Could you check a few things on this model? Use its own coordinates, in mm. A direction names the side the tool comes from. Coordinates: 2 decimals unless noted, no trailing zeros. Write each loop counter-clockwise with the first axis right and the second up, starting at its lowest first coordinate (ties: lowest second). Pieces come first, ordered by that corner, then holes.
```python
from build123d import *

# Parameters (mm, degrees)
BOSS_EXTRUDE1_DEPTH = 25
SHELL8_T            = -2
CUT_EXTRUDE1_DEPTH  = 76
SKETCH3_W           = 98
SKETCH3_H           = 98
CUT_EXTRUDE2_DEPTH  = 2
FILLET1_R           = 2
FILLET2_R           = 2


with BuildPart() as part:
    # Sketch1 → Boss-Extrude1 (new body)
    with BuildSketch(Plane(origin=(0, 0, 0), x_dir=(1, 0, 0), z_dir=(0, 1, 0))):
        Polygon((0, -50), (50, -50), (50, 50), (-50, 50), (-50, -50), align=None)
    extrude(amount=BOSS_EXTRUDE1_DEPTH)

    # Shell8
    shell8_openings = [part.faces().sort_by_distance(p)[0] for p in [
        (0, 25, 0),
    ]]
    offset(amount=SHELL8_T, openings=shell8_openings, kind=Kind.INTERSECTION)

    # Sketch2 → Cut-Extrude1 (cut, through all)
    with BuildSketch(Plane.XY):
        with BuildLine():
            ThreePointArc((3.75, 17.255), (3.58890873, 16.86609127), (3.2, 16.705))
            Line((3.2, 16.705), (-3.2, 16.705))
            ThreePointArc((-3.2, 16.705), (-3.58890873, 16.86609127), (-3.75, 17.255))
            Line((-3.75, 17.255), (-3.75, 18.001446611))
            ThreePointArc((-3.75, 18.001446611), (-3.708133743, 18.211922498), (-3.58890873, 18.390355339))
            Line((-3.58890873, 18.390355339), (-2.985355339, 18.99390873))
            ThreePointArc((-2.985355339, 18.99390873), (-2.806922497, 19.113133743), (-2.596446609, 19.155))
            Line((-2.596446609, 19.155), (2.596446609, 19.155))
            ThreePointArc((2.596446609, 19.155), (2.806922497, 19.113133743), (2.985355339, 18.99390873))
            Line((2.985355339, 18.99390873), (3.58890873, 18.390355339))
            ThreePointArc((3.58890873, 18.390355339), (3.708133743, 18.211922498), (3.75, 18.001446611))
            Line((3.75, 18.001446611), (3.75, 17.255))
        make_face()
    extrude(amount=CUT_EXTRUDE1_DEPTH, mode=Mode.SUBTRACT)

    # Sketch3 → Cut-Extrude2 (cut)
    with BuildSketch(Plane(origin=(0, 25, 0), x_dir=(1, 0, 0), z_dir=(0, 1, 0))):
        Rectangle(SKETCH3_W, SKETCH3_H)
    extrude(amount=-CUT_EXTRUDE2_DEPTH, mode=Mode.SUBTRACT)

    # Fillet1
    fillet1_edges = [part.edges().sort_by_distance(p)[0] for p in [
        (-50, 12.5, 50),
        (-50, 12.5, -50),
        (50, 12.5, -50),
        (50, 12.5, 50),
    ]]
    fillet(fillet1_edges, radius=FILLET1_R)

    # Fillet2
    fillet2_edges = [part.edges().sort_by_distance(p)[0] for p in [
        (-48, 12.5, -48),
        (-48, 12.5, 48),
        (48, 12.5, -48),
        (48, 12.5, 48),
    ]]
    fillet(fillet2_edges, radius=FILLET2_R)


solid = part.part
```
Item 1: Will these pins go through, and if not, where does the flat tip stop? pin 1 Ø1.5 at (x, z) = (1, 7.5) entering from +Y; pin 2 Ø0.8 at (y, z) = (18, 49) entering from -X.
Item 2: I want a section at B-B, the plane z = 34. List the corners of the cut face in (x, y) for me.
Item 3: Which directions (+Z, -Z, +X, -X, +Y, -Y) give clear straight access to the entire face, cutting with the end or side of a thin tool? Please do faces 1 (the flat face through (-1, 12, 48)), 2 (the flat face through (-50, 12, -1)).
Item 4: If I drill on line 1 along Z through (x, y) = (13, 17.5); line 2 along X through (y, z) = (24, 34.5), over which ranges is the centre line in solid material (lowest first)?
Item 5: I want a section at C-C, the plane x = -25.5. List the corners of the cut face in (y, z) for me, then the cut area to 3 significant figures.
Item 6: If we mould it in two halves opening along X, with no side actions, what happens to faces 3 (the flat face through (-1, 0, -1)), 4 (the flat face through (48, 12, 1)), 5 (the flat face through (50, 12, 1))? For each: released by +X, released by -X, zero draft, split by the parting line, or undercut.
Item 7: I want a section at A-A, the plane y = 10. List the corners of the cut face in (x, z) for me.
Taken from the geometry:
1. pin 1: stops at y = 2
1. pin 2: stops at x = -49.91
2. outline: (-50, 0) - (50, 0) - (50, 25) - (49, 25) - (49, 23) - (48, 23) - (48, 2) - (-48, 2) - (-48, 23) - (-49, 23) - (-49, 25) - (-50, 25) - close
3. face 1: +Y
3. face 2: +Z, -Z, -X, +Y, -Y
4. line 1: z = -50 to -48, 48 to 50
4. line 2: x = -50 to -49, 49 to 50
5. outline: (0, -50) - (25, -50) - (25, -49) - (23, -49) - (23, -48) - (2, -48) - (2, 48) - (23, 48) - (23, 49) - (25, 49) - (25, 50) - (0, 50) - close
5. area: 288 mm2
6. face 3: zero draft
6. face 4: undercut
6. face 5: released by +X
7. outline: (-50, -48) arc R2 ccw to (-48, -50) - (48, -50) arc R2 ccw to (50, -48) - (50, 48) arc R2 ccw to (48, 50) - (-48, 50) arc R2 ccw to (-50, 48) - close; hole (-48, -46) arc R2 ccw to (-46, -48) - (46, -48) arc R2 ccw to (48, -46) - (48, 46) arc R2 ccw to (46, 48) - (-46, 48) arc R2 ccw to (-48, 46) - close
